from build123d import *

# Parameters (mm, degrees)
CUT_EXTRUDE_START   = -1.999988779
CUT_EXTRUDE_1_DEPTH = 2.999988779


with BuildPart() as part:
    # Sketch 1 one side → Revolve 2 (revolve)
    with BuildSketch(Plane.XY, mode=Mode.PRIVATE) as revolve_2_sk:
        with BuildLine():
            Line((0, 0), (0, 10))
            Line((0, 10), (-2.16, 10))
            Line((-2.16, 10), (-2.5, 9.66))
            Line((-2.5, 9.66), (-2.5, 0))
            Line((-2.5, 0), (-4.75, 0))
            ThreePointArc((-4.75, 0), (-3.877015605, -1.581194586), (-2.5, -2.75))
            Line((-2.5, -2.75), (-1.5, -2.75))
            Line((-1.5, -2.75), (-1.5, -0.75))
            Line((-1.5, -0.75), (0, 0))
        make_face()
    revolve(revolve_2_sk.sketch.rotate(Axis((0, 0, 0), (0, 1, 0)), 270), axis=Axis((0, 0, 0), (0, 1, 0)))

    # Cut-Extrude 1: read off the stored shape, not the designer's step
    # Cut-Extrude 1 outline → Cut-Extrude 1 (cut)
    with BuildSketch(Plane.XZ.offset(2.75).offset(CUT_EXTRUDE_START)):
        with BuildLine():
            Line((0, -1.5), (0.866025404, -1.5))
            Line((0.866025404, -1.5), (1.29903811, -0.749999993))
            ThreePointArc((1.29903811, -0.749999993), (0.750000003, -1.299038104), (0, -1.5))
        make_face()
        with BuildLine():
            ThreePointArc((1.299038111, 0.749999991), (1.5, -1e-09), (1.29903811, -0.749999993))
            Line((1.29903811, -0.749999993), (1.732050808, 0))
            Line((1.732050808, 0), (1.299038111, 0.749999991))
        make_face()
        with BuildLine():
            Line((-0.866025404, -1.5), (0, -1.5))
            ThreePointArc((0, -1.5), (-0.750000001, -1.299038105), (-1.299038107, -0.749999998))
            Line((-1.299038107, -0.749999998), (-0.866025404, -1.5))
        make_face()
        with BuildLine():
            Line((-1.732050808, 0), (-1.299038107, -0.749999998))
            ThreePointArc((-1.299038107, -0.749999998), (-1.5, 2e-09), (-1.299038105, 0.750000001))
            Line((-1.299038105, 0.750000001), (-1.732050808, 0))
        make_face()
        with BuildLine():
            ThreePointArc((0, 1.5), (0.750000004, 1.299038103), (1.299038111, 0.749999991))
            Line((1.299038111, 0.749999991), (0.866025404, 1.5))
            Line((0.866025404, 1.5), (0, 1.5))
        make_face()
        with BuildLine():
            Line((-0.866025404, 1.5), (-1.299038105, 0.750000001))
            ThreePointArc((-1.299038105, 0.750000001), (-0.75, 1.299038106), (0, 1.5))
            Line((0, 1.5), (-0.866025404, 1.5))
        make_face()
    extrude(amount=CUT_EXTRUDE_1_DEPTH, mode=Mode.SUBTRACT)

    # Cut-Extrude 1 2 outline → Cut-Extrude 1 2 (revolve)
    with BuildSketch(Plane.XY):
        Polygon((1.732050808, -0.750011221), (1.5, -0.750011221), (1.732050812, -0.866025406), align=None)
    revolve(axis=Axis((0, 0, 0), (0, 1, 0)))


solid = part.part
Could you check a few things on this model? Use its own coordinates, in mm. A direction names the side the tool comes from. Give positions to 0.01 mm unless a question says otherwise; leave off trailing zeros. Order: outer loops, then holes, each group sorted by start corner. A loop starts at its lowest first (then second) coordinate and runs counter-clockwise, first axis right, second up.
1. Which directions (+Z, -Z, +X, -X, +Y, -Y) give clear straight access to the entire face, cutting with the end or side of a thin tool? Please do faces 4 (the flat face through (0, -2.75, -2)), 5 (the flat face through (0, -2, 1.5)).
Answers below:
face 4: +Z, -Z, +X, -X, -Y
face 5: -Y
2. Suppose I cut it at A-A (y = -1.5). Write out the boundary of the cut face in (x, z), plus the area to 3 significant figures.
Answers below:
outline: circle Ø7.88 at (0, 0); hole (-1.73, 0) - (-0.87, -1.5) - (0.87, -1.5) - (1.73, 0) - (0.87, 1.5) - (-0.87, 1.5) - close
area: 41.0 mm2
3. Suppose I cut it at D-D (z = 3.5). Write out the boundary of the cut face in (x, y), plus the area to 3 significant figures.
Answers below:
outline: (-3.21, 0) arc R3.58 ccw to (3.21, 0) - close
area: 9.16 mm2
4. Suppose I cut it at C-C (x = 3.5). Write out the boundary of the cut face in (y, z).
Answers below:
outline: (0, -3.21) - (0, 3.21) arc R3.58 ccw to start
5. I need wall thicknesses on L1, parallel to Z at x = 2, y = 3.25; L2, parallel to Y at x = 1, z = 2.75; L3, parallel to Y at x = 1.5, z = -3.5. Which ranges of each line are inside material? Lowest first, please.
Answers below:
L1: z = -1.5 to 1.5
L2: y = -2.47 to 0
L3: y = -1.66 to 0
6. For pin 1 (1.9 mm diameter, centred on x = 0, y = -1.5, fed in from -Z); pin 2 (5 mm diameter, centred on y = 5, z = 2.5, fed in from -X); pin 3 (5 mm diameter, centred on x = 0.5, y = 4.5, fed in from +Z), each with a flat end and sliding along its axis, tell me the tip position at first contact or that it passes through.
Answers below:
pin 1: stops at z = -4.53
pin 2: stops at x = -2.5
pin 3: stops at z = 2.5
7. Thinking about a two-plate mould opening in X: for faces 1 (the flat face through (2, 0, 2)), 2 (the flat face through (0, -2, -1.5)), 3 (the cylindrical face through (2.44, 4.76, 0.54)), which applies, +X half, -X half, draft (parallel to the pull), parting line (faces both ways), or undercut?
Answers below:
face 1: draft
face 2: undercut
face 3: parting line
8. Suppose I cut it at B-B (y = 6.75). Write out the boundary of the cut face in (x, z), plus the area to 3 significant figures.
Answers below:
outline: circle Ø5 at (0, 0)
area: 19.6 mm2
